Verification items for the finished model (mm, model axes). A direction names the side the tool comes from. Round coordinates to 2 decimals unless told otherwise and drop trailing zeros. Write each loop counter-clockwise with the first axis right and the second up, starting at its lowest first coordinate (ties: lowest second). Pieces come first, ordered by that corner, then holes. Notation, with made-up numbers: (3, 6) - (54, 6) arc R20 ccw to (54, 26) - close; hole circle Ø10 at (21.25, -22.5). An arc over 180 degrees is marked (long way). Answer as a JSON object with one key per item and string values.
```python
from build123d import *

# Parameters (mm, degrees)
SKETCH2_R                = 48.5
BOSS_EXTRUDE1_DEPTH      = 4
SKETCH4_R                = 1.5
CUT_EXTRUDE2_DEPTH       = 5
SKETCH5_R                = 3.75
CUT_EXTRUDE3_DEPTH       = 1.5
BOSS_EXTRUDE2_DEPTH      = 14
CUT_EXTRUDE5_REACH       = 44.5
SKETCH9_R                = 1.3
CUT_EXTRUDE6_DEPTH       = 7.5
CUT_EXTRUDE9_REACH       = 46.5
SKETCH11_R               = 9
BOSS_EXTRUDE7_DEPTH      = 9
BOSS_EXTRUDE7_DEPTH_BACK = 14
BOSS_EXTRUDE10_DEPTH     = 9
SKETCH27_W               = 16
SKETCH27_H               = 6
BOSS_EXTRUDE11_DEPTH     = 12
FILLET6_R                = 3
CUT_EXTRUDE16_REACH      = 75.05
SKETCH28_W               = 8
SKETCH28_H               = 4
CUT_EXTRUDE17_DEPTH      = 49.5
CUT_EXTRUDE17_DEPTH_BACK = 49.5


with BuildPart() as part:
    # Sketch2 → Boss-Extrude1 (new body)
    with BuildSketch(Plane(origin=(0, 0, 0), x_dir=(1, 0, 0), z_dir=(0, 1, 0))):
        Circle(SKETCH2_R)
    extrude(amount=BOSS_EXTRUDE1_DEPTH)

    # Sketch4 → Cut-Extrude2 (cut, through all)
    with BuildSketch(Plane.XZ):
        with Locations((0, 7.25)):
            Circle(SKETCH4_R)
        with Locations((0, -7.25)):
            Circle(SKETCH4_R)
    extrude(amount=-CUT_EXTRUDE2_DEPTH, mode=Mode.SUBTRACT)

    # Sketch5 → Cut-Extrude3 (cut)
    with BuildSketch(Plane.XZ):
        Circle(SKETCH5_R)
    extrude(amount=-CUT_EXTRUDE3_DEPTH, mode=Mode.SUBTRACT)

    # Sketch7 → Boss-Extrude2 (add)
    with BuildSketch(Plane(origin=(-4, 0, 0), x_dir=(0, 0, -1), z_dir=(1, 0, 0))):
        with BuildLine():
            Line((23.129947874, 4), (23.129947874, 11.644549616))
            ThreePointArc((23.129947874, 11.644549616), (24.589048403, 18.743749901), (28.729797284, 24.692011643))
            ThreePointArc((28.729797284, 24.692011643), (29.313383054, 55.284736897), (-1.284289494, 55.479275971))
            Line((-1.284289494, 55.479275971), (-27.227315747, 29.536249718))
            ThreePointArc((-27.227315747, 29.536249718), (-32.64663453, 21.425665997), (-34.549646217, 11.858580188))
            Line((-34.549646217, 11.858580188), (-34.549646217, 4))
            Line((-34.549646217, 4), (23.129947874, 4))
        make_face()
    extrude(amount=-BOSS_EXTRUDE2_DEPTH)

    # Sketch8 → Cut-Extrude5 (cut, up to next)
    with BuildSketch(Plane(origin=(-6, 0, 0), x_dir=(0, 0, -1), z_dir=(1, 0, 0)), mode=Mode.PRIVATE) as cut_extrude5_sk1:
        Polygon((-15.249648422, 25.957567857), (13.741729607, 54.948945886), (28.590972012, 40.099703481), (-0.400406017, 11.108325452), align=None)
    cut_extrude5_tool1 = extrude(cut_extrude5_sk1.sketch, amount=-CUT_EXTRUDE5_REACH, mode=Mode.PRIVATE) & part.part
    add(cut_extrude5_tool1.solids().sort_by_distance((-6, 33.028636, -6.670662))[0], mode=Mode.SUBTRACT)

    # Sketch9 → Cut-Extrude6 (cut)
    with BuildSketch(Plane.ZY.offset(18)):
        with Locations((-20.105690637, 53.534732323)):
            Circle(SKETCH9_R)
        with Locations((-27.176758449, 46.463664511)):
            Circle(SKETCH9_R)
        with Locations((6.764367048, 12.522539014)):
            Circle(SKETCH9_R)
        with Locations((13.83543486, 19.593606826)):
            Circle(SKETCH9_R)
    extrude(amount=-CUT_EXTRUDE6_DEPTH, mode=Mode.SUBTRACT)

    # Sketch11 → Cut-Extrude9 (cut, up to next)
    with BuildSketch(Plane(origin=(-4, 0, 0), x_dir=(0, 0, -1), z_dir=(1, 0, 0)), mode=Mode.PRIVATE) as cut_extrude9_sk1:
        with Locations((13.918506302, 40.276480176)):
            Circle(SKETCH11_R)
    cut_extrude9_tool1 = extrude(cut_extrude9_sk1.sketch, amount=-CUT_EXTRUDE9_REACH, mode=Mode.PRIVATE) & part.part
    add(cut_extrude9_tool1.solids().sort_by_distance((-4, 40.27648, -13.918506))[0], mode=Mode.SUBTRACT)

    # Sketch17 → Boss-Extrude7 (add, two sides)
    with BuildSketch(Plane.ZY.offset(18)) as boss_extrude7_sk:
        with BuildLine():
            ThreePointArc((34.549646217, 11.858580188), (33.008342843, 20.500891953), (28.574482006, 28.077569775))
            ThreePointArc((28.574482006, 28.077569775), (27.915386359, 28.820289685), (27.227315747, 29.536249718))
            Line((27.227315747, 29.536249718), (1.284289494, 55.479275971))
            Line((1.284289494, 55.479275971), (26.295003593, 26.127182305))
            ThreePointArc((26.295003593, 26.127182305), (30.194232218, 19.461281607), (31.549646217, 11.858580188))
            Line((31.549646217, 11.858580188), (31.549646217, 4))
            Line((31.549646217, 4), (34.549646217, 4))
            Line((34.549646217, 4), (34.549646217, 11.858580188))
        make_face()
        with BuildLine():
            Line((28.574482006, 28.077569775), (3.405609837, 57.600596315))
            ThreePointArc((3.405609837, 57.600596315), (-31.461505391, 57.378912253), (-30.796489049, 22.517434639))
            ThreePointArc((-30.796489049, 22.517434639), (-27.345864981, 17.560549854), (-26.129947874, 11.644549616))
            Line((-26.129947874, 11.644549616), (-26.129947874, 4))
            Line((-26.129947874, 4), (-23.129947874, 4))
            Line((-23.129947874, 4), (-23.129947874, 11.644549616))
            ThreePointArc((-23.129947874, 11.644549616), (-24.589048403, 18.743749901), (-28.729797284, 24.692011643))
            ThreePointArc((-28.729797284, 24.692011643), (-29.313383054, 55.284736897), (1.284289494, 55.479275971))
            Line((1.284289494, 55.479275971), (27.227315747, 29.536249718))
            ThreePointArc((27.227315747, 29.536249718), (27.915386359, 28.820289685), (28.574482006, 28.077569775))
        make_face()
    extrude(amount=BOSS_EXTRUDE7_DEPTH)
    extrude(boss_extrude7_sk.sketch, amount=-BOSS_EXTRUDE7_DEPTH_BACK)

    # Sketch25 → Boss-Extrude10 (add)
    with BuildSketch(Plane.ZY.offset(18)):
        with BuildLine():
            ThreePointArc((-28.729797284, 24.692011643), (-24.589048403, 18.743749901), (-23.129947874, 11.644549616))
            Line((-23.129947874, 11.644549616), (-23.129947874, 4))
            Line((-23.129947874, 4), (-15.129947874, 4))
            add(Edge.make_bspline(
                [(-28.729797284, 24.692011643), (-21.954867515, 18.253200081), (-19.09405247, 12.798017691), (-15.129947874, 4)],
                knots=[0, 0, 0, 0, 1, 1, 1, 1], degree=3))
        make_face()
        with BuildLine():
            add(Edge.make_bspline(
                [(11.751619577, 43.19501844), (26.551255916, 25.8264495), (25.549646217, 4)],
                knots=[0, 0, 0, 1, 1, 1], degree=2))
            Line((25.549646217, 4), (31.549646217, 4))
            Line((31.549646217, 4), (31.549646217, 11.858580188))
            ThreePointArc((31.549646217, 11.858580188), (30.194232218, 19.461281607), (26.295003593, 26.127182305))
            Line((26.295003593, 26.127182305), (11.751619577, 43.19501844))
        make_face()
    extrude(amount=BOSS_EXTRUDE10_DEPTH)

    # Sketch27 → Boss-Extrude11 (add)
    with BuildSketch(Plane(origin=(0, 4, 0), x_dir=(1, 0, 0), z_dir=(0, 1, 0))):
        with Locations((6, -21.549646217)):
            Rectangle(SKETCH27_W, SKETCH27_H)
    extrude(amount=BOSS_EXTRUDE11_DEPTH)

    # Fillet6
    fillet6_edges = [part.edges().sort_by_distance(p)[0] for p in [
        (-2, 16, 21.549646217),
        (14, 16, 21.549646217),
    ]]
    fillet(fillet6_edges, radius=FILLET6_R)

    # Sketch28 → Cut-Extrude16 (cut, up to next)
    with BuildSketch(Plane.XY.offset(24.549646217), mode=Mode.PRIVATE) as cut_extrude16_sk1:
        with Locations((6, 10)):
            Rectangle(SKETCH28_W, SKETCH28_H)
    cut_extrude16_tool1 = extrude(cut_extrude16_sk1.sketch, amount=-CUT_EXTRUDE16_REACH, mode=Mode.PRIVATE) & part.part
    add(cut_extrude16_tool1.solids().sort_by_distance((6, 10, 24.549646))[0], mode=Mode.SUBTRACT)

    # Sketch29 → Cut-Extrude17 (cut, two sides)
    with BuildSketch(Plane.XY) as cut_extrude17_sk:
        with BuildLine():
            Line((-21, 64.776480176), (-27, 64.776480176))
            Line((-27, 64.776480176), (-27, 4))
            Line((-27, 4), (-26.5, 4))
            add(Edge.make_bspline(
                [(-21, 64.776480176), (-21.220459696, 34.140901434), (-26.5, 4)],
                knots=[0, 0, 0, 1, 1, 1], degree=2))
        make_face()
    extrude(amount=CUT_EXTRUDE17_DEPTH, mode=Mode.SUBTRACT)
    extrude(cut_extrude17_sk.sketch, amount=-CUT_EXTRUDE17_DEPTH_BACK, mode=Mode.SUBTRACT)


solid = part.part
```
1. Cross-section at C-C (x = -41). Record the boundary of the cut face in (y, z), plus the area to 3 significant figures.
Completed:
{"outline": "(0, -25.91) - (4, -25.91) - (4, 25.91) - (0, 25.91) - close", "area": "207 mm^2"}
2. Go/stop test with flat-tipped pins: pin 1 (8.5 mm diameter, centred on x = -18, y = 6, fed in from -Z); pin 2 (3.5 mm diameter, centred on y = 19.59, z = 13.84, fed in from +X); pin 3 (0.8 mm diameter, centred on y = 46, z = -27, fed in from -X); pin 4 (1.8 mm diameter, centred on x = 0, z = -7.25, fed in from +Y). Record where each tip stops, or that it passes through.
Completed:
{"pin 1": "stops at z = -46.36", "pin 2": "stops at x = -4", "pin 3": "stops at x = -10.5", "pin 4": "passes through"}
3. Access from +Z, -Z, +X, -X, +Y, -Y to the whole of each face (thin tool, end or side, straight path). Record for faces 1 (the face through (-2, 8, 22)), 2 (the face through (-15, 8, -26.13)), 3 (the face through (-20.092, 48.622, -33.733)).
Completed:
{"face 1": "+Z, -Z, +Y", "face 2": "-Z, +X, -X", "face 3": "-X"}
4. Mould release check, pull along X, two halves, no side actions. Record for faces 4 (the face through (-14.302, 20.69, 14.534)), 5 (the face through (-1.14, 15.1, 21.51)), 6 (the face through (14, 8, 22)): released by +X, released by -X, zero draft, split by the parting line, or undercut.
Completed:
{"face 4": "zero draft", "face 5": "undercut", "face 6": "released by +X"}
5. Cross-section at B-B (z = -7.25). Count the separate pieces of the cut face and the enclosed holes in it, plus the area to 3 significant figures.
Completed:
{"separate pieces": "3", "enclosed holes": "0", "area": "838 mm^2"}
6. Cross-section at D-D (x = 36.5). Record the boundary of the cut face in (y, z).
Completed:
{"outline": "(0, -31.94) - (4, -31.94) - (4, 31.94) - (0, 31.94) - close"}
7. Cross-section at A-A (x = -14.5). Record the boundary of the cut face in (y, z), plus the area to 3 significant figures.
Completed:
{"outline": "(0, -46.28) - (4, -46.28) - (4, -26.13) - (11.64, -26.13) arc R15 cw to (22.52, -30.8) arc R24.5 ccw (long way) to (57.6, 3.41) - (28.08, 28.57) arc R25 ccw to (11.86, 34.55) - (4, 34.55) - (4, 46.28) - (0, 46.28) - close; hole (11.11, 0.4) - (40.1, -28.59) - (54.95, -13.74) - (25.96, 15.25) - close; hole circle Ø2.6 at (12.52, 6.76); hole circle Ø2.6 at (19.59, 13.84); hole circle Ø2.6 at (46.46, -27.18); hole circle Ø2.6 at (53.53, -20.11)", "area": "2,700 mm^2"}
8. Material ranges on probe 1 along Z at (x, y) = (0, 1.05); probe 2 along Y at (x, z) = (0, -16); probe 3 along Z at (x, y) = (13.5, 13.5), recorded low to high. Write a range as from..to.
Completed:
{"probe 1": "z = -48.5..-8.75, -5.75..-3.75, 3.75..5.75, 8.75..48.5", "probe 2": "y = 0..4", "probe 3": "z = 18.55..24.55"}
